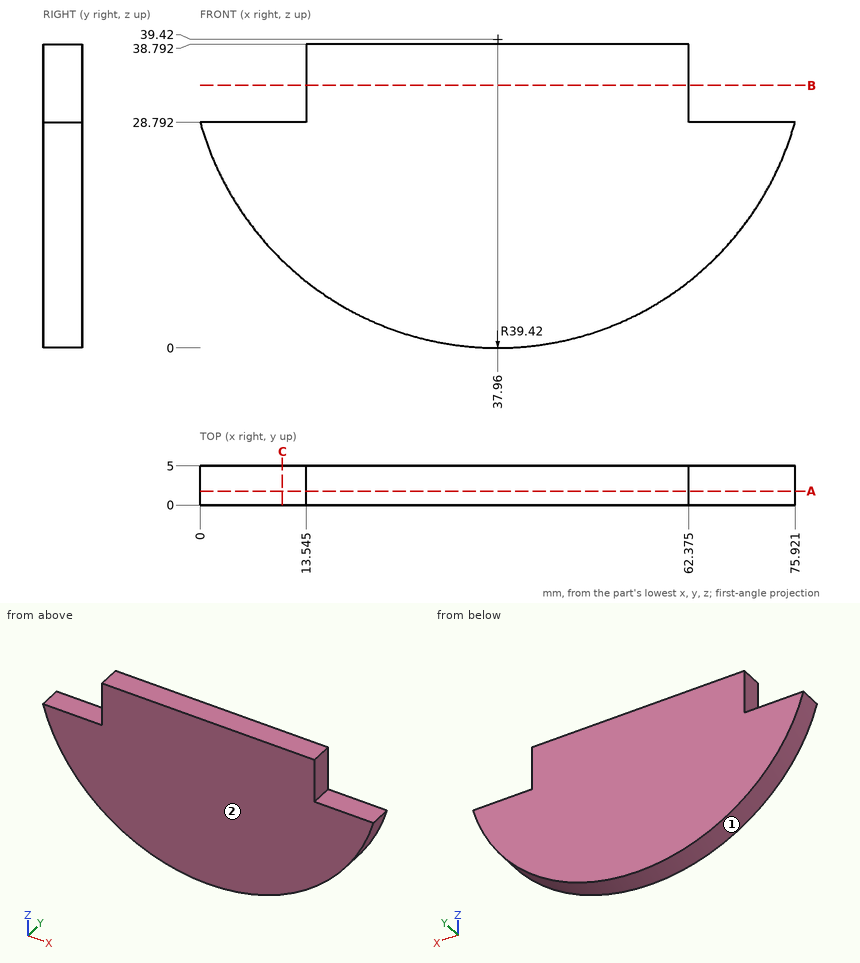
Source: three-view drawing plus pictorial views. Frame: mm from the lowest corner of the part. Coordinates: 2 decimals unless noted, no trailing zeros. Loops run counter-clockwise (first coordinate to the right, second up) from the corner with the lowest first, then second, coordinate; pieces in that order, holes last. Notation, with made-up numbers: M 44.25,78 L 55.25,78 A33 ccw 55.25,111 Z; hole C 56,42 d4. An arc over 180 degrees is marked long. Use CSV: the item, a comma, the result in double quotes.
(1) Cut plane B-B on z = 33.5. Return loops of the section in (x, y) (1 decimal).
Answers follow:
outline,"M 13.5,0 L 62.4,0 L 62.4,5 L 13.5,5 Z"
(2) Draft query along X for the marked faces 1 and 2. Return one class per face: pulls with the +X half, pulls with the -X half, needs draft (parallel to the pull), parting line crosses it, or undercut.
Answers follow:
face 1,"parting line crosses it"
face 2,"needs draft"
(3) Line query: line 1 (Z direction, x = 37, y = 1.3); line 2 (X direction, y = 1, z = 29) (1 decimal); line 3 (Z direction, x = 8.5, y = 1.9). Output: solid intervals per line, ascending. Write a range as [from, to].
Answers follow:
line 1,"[0.01, 38.79]"
line 2,"[13.5, 62.4]"
line 3,"[13.23, 28.79]"
(4) Cut plane A-A on y = 1.8. Return loops of the section in (x, z) (1 decimal).
Answers follow:
outline,"M 0,28.8 A39.4 ccw 75.9,28.8 L 62.4,28.8 L 62.4,38.8 L 13.5,38.8 L 13.5,28.8 Z"
(5) Cut plane C-C on x = 10.5. Return loops of the section in (y, z).
Answers follow:
outline,"M 0,11.14 L 5,11.14 L 5,28.79 L 0,28.79 Z"
(6) Contact query for flat-ended pins moving along their axis: pin 1 (2.5 mm diameter, centred on x = 3.5, y = 3.5, fed in from +Z); pin 2 (3 mm diameter, centred on y = 1.5, z = 31, fed in from +X) (1 decimal); pin 3 (2 mm diameter, centred on y = 1.5, z = 9.5, fed in from -X). Output: stop coordinate, or through.
Answers follow:
pin 1,"z = 28.79"
pin 2,"x = 62.4"
pin 3,"x = 11.17"
